The drawing under review shows one solid part. Ordinate dimensions are in mm from its lowest x, y, z. A direction names the side the tool comes from. Coordinates: 2 decimals unless noted, no trailing zeros. Order: outer loops, then holes, each group sorted by start corner. A loop starts at its lowest first (then second) coordinate and runs counter-clockwise, first axis right, second up. Notation, with made-up numbers: (88, -13.5) -> (100, -13.5) arc R19 cw to (100, 0.5) -> close; hole circle Ø6 at (13, 82). An arc over 180 degrees is marked (long way). Write item = value, one per line.
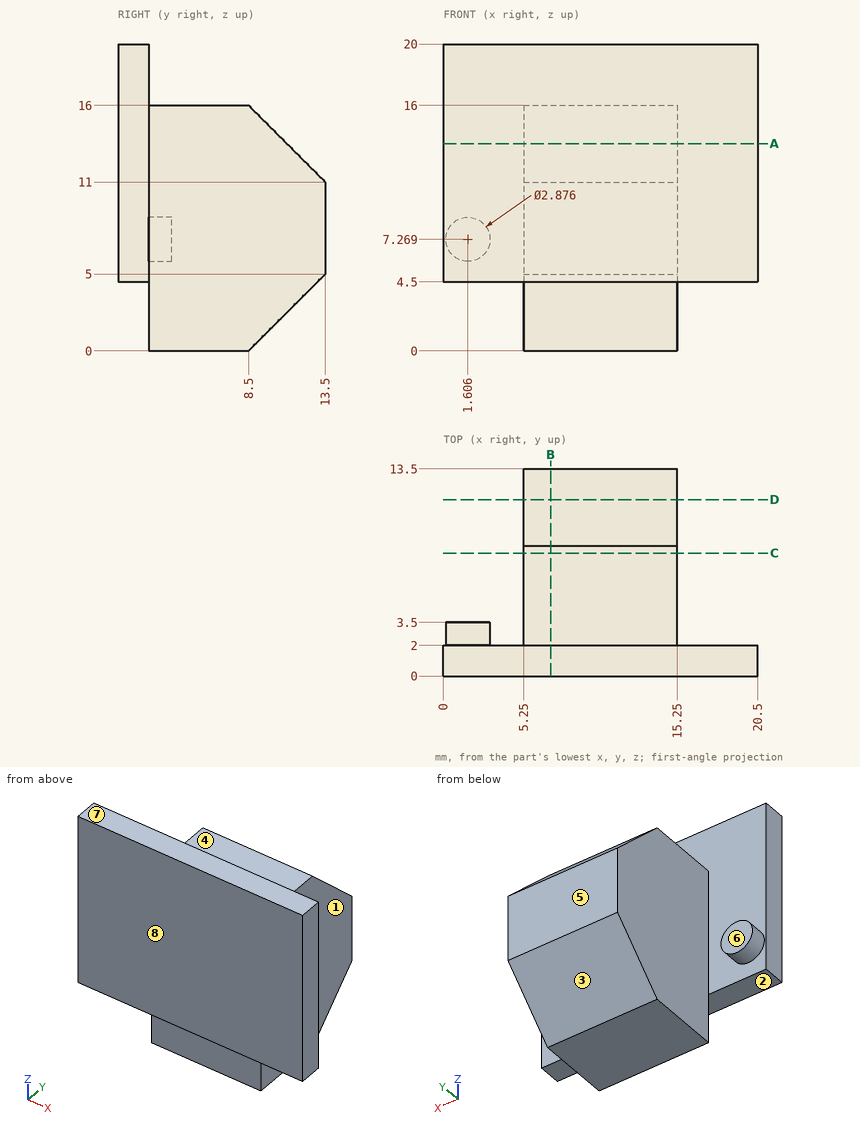
(1) The part is to be moulded in two halves that separate along Y. For the marked faces 6, 7 and 8, say which applies: released by +Y, released by -Y, zero draft, split by the parting line, or undercut.
Report:
face_6 = released by +Y
face_7 = zero draft
face_8 = released by -Y
(2) For the marked faces 1, 2, 3, 4 and 5, list the 3-axis set-ups (+Z, -Z, +X, -X, +Y, -Y) from which the entire face can be reached by the end or side of a thin tool; tool diameter is ignored.
Report:
face_1 = +Z, -Z, +X, +Y
face_2 = -Z, +X, -X, -Y
face_3 = -Z, +X, -X, +Y
face_4 = +Z, +X, -X, +Y
face_5 = +Z, -Z, +X, -X, +Y
(3) We need section C-C (y = 8). Write out the cut boundary in (x, z).
Report:
outline = (5.25, 0) -> (15.25, 0) -> (15.25, 16) -> (5.25, 16) -> close
(4) We need section D-D (y = 11.5). Write out the cut boundary in (x, z), and give its area (4 significant figures).
Report:
outline = (5.25, 3) -> (15.25, 3) -> (15.25, 13) -> (5.25, 13) -> close
area = 100.0 mm²
(5) We need section B-B (x = 7). Write out the cut boundary in (y, z).
Report:
outline = (0, 4.5) -> (2, 4.5) -> (2, 0) -> (8.5, 0) -> (13.5, 5) -> (13.5, 11) -> (8.5, 16) -> (2, 16) -> (2, 20) -> (0, 20) -> close
(6) We need section A-A (z = 13.5). Write out the cut boundary in (x, y).
Report:
outline = (0, 0) -> (20.5, 0) -> (20.5, 2) -> (15.25, 2) -> (15.25, 11) -> (5.25, 11) -> (5.25, 2) -> (0, 2) -> close
(7) Insertion check: pin 1 (1.5 mm diameter, centred on x = 9, z = 14, fed in from +Y); pin 2 (3 mm diameter, centred on y = 5.5, z = 15.5, fed in from +X); pin 3 (5 mm diameter, centred on y = 12, z = 15.5, fed in from -X); pin 4 (6 mm diameter, centred on x = 16.5, z = 13.5, fed in from +Y). Each pin has a flat end and moves straight along its axis. Give the tip position at first contact, or say it passes through.
Report:
pin_1 = 11.25
pin_2 = 15.25
pin_3 = 5.25
pin_4 = 13.5
(8) For L1, parallel to X at y = 8.5, z = 11.75; L2, parallel to Z at x = 11.5, y = 1; L3, parallel to Y at x = 1.5, z = 11, list the stretches that pass through material, from the lowest coordinate up.
Report:
L1 = 5.25 to 15.25
L2 = 4.5 to 20
L3 = 0 to 2
